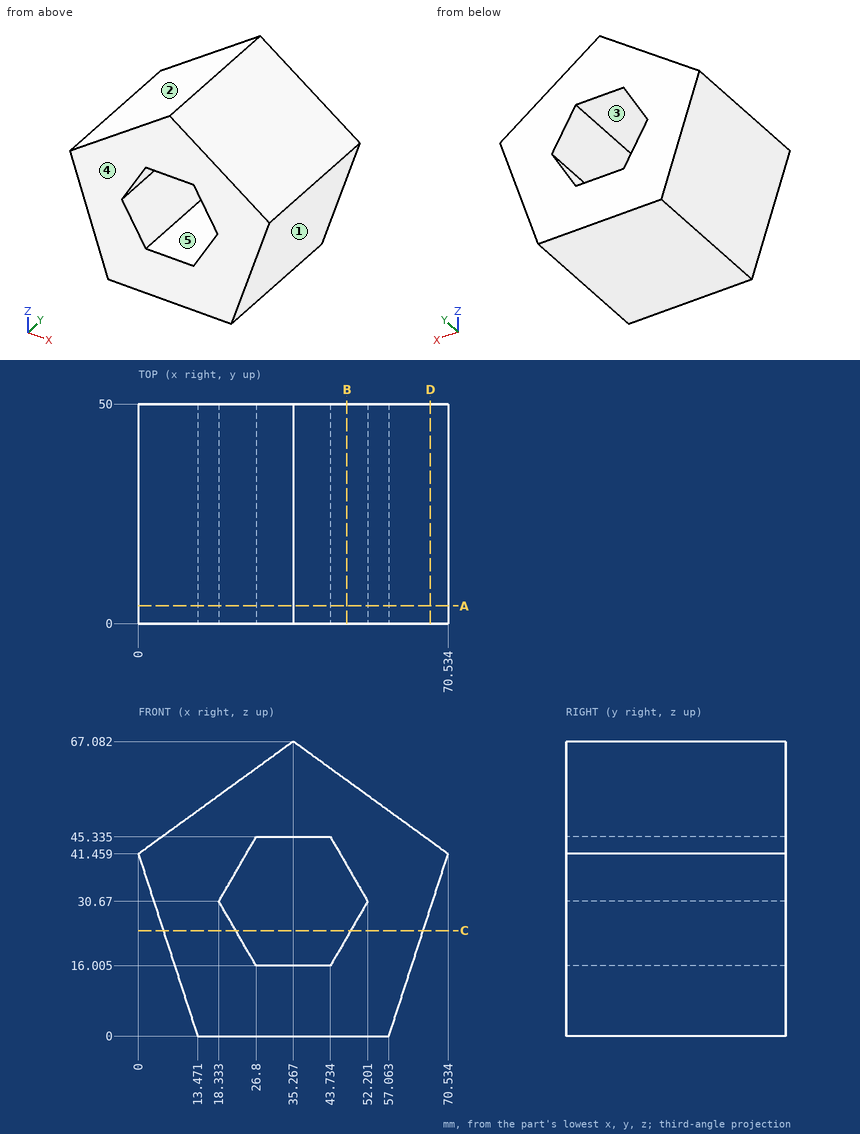
Geometry check sheet. Reference: drawing and pictorial views, mm from the part's lowest x, y, z. A direction names the side the tool comes from. Coordinates: 2 decimals unless noted, no trailing zeros. Order: outer loops, then holes, each group sorted by start corner. A loop starts at its lowest first (then second) coordinate and runs counter-clockwise, first axis right, second up. Notation, with made-up numbers: (85.5, 38.5) -> (126.5, 38.5) arc R17 cw to (126.5, 57.5) -> close; hole circle Ø7 at (48, 62.5). An arc over 180 degrees is marked (long way). Use CSV: the item, a comma, the result in double quotes. Start each with the question number.
Q1. Tool access check on the marked faces 4 and 5. Record the directions out of +Z, -Z, +X, -X, +Y, -Y that give a thin tool (end or side, any length) a straight path to the whole face; none if there is none.
Q2. Section check A-A, the plane y = 4. Record the cut outline in (x, z) (1 decimal), and give its area (3 significant figures).
Q3. Section check C-C, the plane z = 24. Record the cut outline in (x, y).
Q4. Section check D-D, the plane x = 66.5. Record the cut outline in (y, z).
Q5. Section check B-B, the plane x = 47.5. Record the cut outline in (y, z) (1 decimal), and give its area (3 significant figures).
Q6. Depth check by flat-ended pin: P1, Ø12, axis at y = 38, z = 23, coming from the -X side; P2, Ø6, axis at x = 48.5, y = 11.5, coming from the +Z side; P3, Ø5, axis at x = 33.5, y = 36.5, coming from the +Z side. Enter the tip coordinate at first touch or a pass-through.
Q7. Draft check along Z on the marked faces 1, 2 and 3. Enter one of: +Z half, -Z half, draft (parallel to the pull), parting line (faces both ways), or undercut.
Q8. Thickness scan on line 1 along Z through (x, y) = (34.5, 24) (1 decimal); line 2 along Z through (x, y) = (47, 6.5) (1 decimal); line 3 along X through (y, z) = (17.5, 30) (1 decimal). Record the ranges inside material, lowest first.
Returned:
1,face 4,"+Z, -Z, +X, -X, -Y"
1,face 5,"+Y, -Y"
2,outline,"(0, 41.5) -> (13.5, 0) -> (57.1, 0) -> (70.5, 41.5) -> (35.3, 67.1) -> close; hole (18.3, 30.7) -> (26.8, 16) -> (43.7, 16) -> (52.2, 30.7) -> (43.7, 45.3) -> (26.8, 45.3) -> close"
2,area,"2,520 mm^2"
3,outline,"(5.67, 0) -> (22.18, 0) -> (22.18, 50) -> (5.67, 50) -> close; (48.35, 0) -> (64.86, 0) -> (64.86, 50) -> (48.35, 50) -> close"
4,outline,"(0, 29.04) -> (50, 29.04) -> (50, 44.39) -> (0, 44.39) -> close"
5,outline,"(0, 0) -> (50, 0) -> (50, 22.5) -> (0, 22.5) -> close; (0, 38.8) -> (50, 38.8) -> (50, 58.2) -> (0, 58.2) -> close"
5,area,"2,100 mm^2"
6,P1,"stops at x = 4.05"
6,P2,"stops at z = 59.65"
6,P3,"stops at z = 67.08"
7,face 1,"-Z half"
7,face 2,"+Z half"
7,face 3,"undercut"
8,line 1,"z = 0 to 16, 45.3 to 66.5"
8,line 2,"z = 0 to 21.7, 39.7 to 58.6"
8,line 3,"x = 3.7 to 18.7, 51.8 to 66.8"
